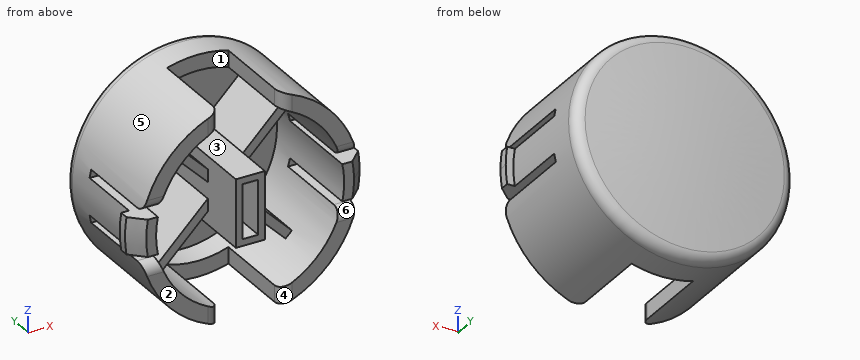
from build123d import *

# Parameters (mm, degrees)
SKETCH2_W     = 6.985
SKETCH2_H     = 32.356336156
SKETCH2_W_2   = 40.972237954
SKETCH2_H_2   = 0.889
CUTOUT_DEPTH  = 10.16
TAB_DEPTH     = 2.54
TAB_CHMF_SIZE = 1.524
CROSS_DEPTH   = 7.62
SKETCH4_W     = 3.302
SKETCH4_H     = 7.6962
BOX_DEPTH     = 13.059399
SKETCH6_W     = 1.778
SKETCH6_H     = 6.1722
BOXCUT_DEPTH  = 13.059399
FILLET1_R     = 1.27


with BuildPart() as part:
    # Sketch1 → dome/base (revolve)
    with BuildSketch(Plane.XY):
        with BuildLine():
            Line((0, 6.039891065), (0, 3.960890157))
            Line((0, 3.960890157), (10.6934, 3.960890157))
            Line((10.6934, 3.960890157), (10.6934, -9.047708935))
            Line((10.6934, -9.047708935), (12.4714, -9.047708935))
            Line((12.4714, -9.047708935), (12.4714, 4.195604597))
            ThreePointArc((12.4714, 4.195604597), (12.144228327, 5.046471653), (11.33128229, 5.45894564))
            ThreePointArc((11.33128229, 5.45894564), (5.673082405, 5.894559394), (0, 6.039891065))
        make_face()
    revolve(axis=Axis((0, 0, 0), (0, 1, 0)))

    # Sketch2 → cutout (cut)
    with BuildSketch(Plane.XZ.offset(9.047708935)):
        Rectangle(SKETCH2_W, SKETCH2_H)
        with Locations((0, 2.54)):
            Rectangle(SKETCH2_W_2, SKETCH2_H_2)
        with Locations((0, -2.54)):
            Rectangle(SKETCH2_W_2, SKETCH2_H_2)
    extrude(amount=-CUTOUT_DEPTH, mode=Mode.SUBTRACT)

    # Sketch3 → tab (add)
    with BuildSketch(Plane.XZ.offset(9.047708935)):
        with BuildLine():
            Line((-13.169324385, -2.0955), (-12.294091984, -2.0955))
            ThreePointArc((-12.294091984, -2.0955), (-12.4714, 0), (-12.294091984, 2.0955))
            Line((-12.294091984, 2.0955), (-13.169324385, 2.0955))
            ThreePointArc((-13.169324385, 2.0955), (-13.335, 0), (-13.169324385, -2.0955))
        make_face()
        with BuildLine():
            Line((12.294091984, -2.0955), (13.169324385, -2.0955))
            ThreePointArc((13.169324385, -2.0955), (13.293516571, -1.051019583), (13.335, 0))
            ThreePointArc((13.335, 0), (13.293516571, 1.051019583), (13.169324385, 2.0955))
            Line((13.169324385, 2.0955), (12.294091984, 2.0955))
            ThreePointArc((12.294091984, 2.0955), (12.4714, 0), (12.294091984, -2.0955))
        make_face()
    extrude(amount=-TAB_DEPTH)

    # tab chmf
    tab_chmf_edges = [part.edges().sort_by_distance(p)[0] for p in [
        (-13.335, -9.047708935, 0),
        (13.335, -9.047708935, 0),
    ]]
    chamfer(tab_chmf_edges, length=TAB_CHMF_SIZE)

    # Sketch5 → cross (add)
    with BuildSketch(Plane.XZ.offset(-3.960890157)):
        with BuildLine():
            Line((0, -0.71842049), (-0.71842049, 0))
            Line((-0.71842049, 0), (-7.91204877, -7.19362828))
            ThreePointArc((-7.91204877, -7.19362828), (-7.561375654, -7.561375654), (-7.19362828, -7.91204877))
            Line((-7.19362828, -7.91204877), (0, -0.71842049))
        make_face()
        with BuildLine():
            Line((7.91204877, -7.19362828), (0.71842049, 0))
            Line((0.71842049, 0), (0, -0.71842049))
            Line((0, -0.71842049), (7.19362828, -7.91204877))
            ThreePointArc((7.19362828, -7.91204877), (7.561375654, -7.561375654), (7.91204877, -7.19362828))
        make_face()
        with BuildLine():
            Line((7.19362828, 7.91204877), (0, 0.71842049))
            Line((0, 0.71842049), (0.71842049, 0))
            Line((0.71842049, 0), (7.91204877, 7.19362828))
            ThreePointArc((7.91204877, 7.19362828), (7.561375654, 7.561375654), (7.19362828, 7.91204877))
        make_face()
        Polygon((0.71842049, 0), (0, 0.71842049), (-0.71842049, 0), (0, -0.71842049), align=None)
        with BuildLine():
            Line((-0.71842049, 0), (0, 0.71842049))
            Line((0, 0.71842049), (-7.19362828, 7.91204877))
            ThreePointArc((-7.19362828, 7.91204877), (-7.561375654, 7.561375654), (-7.91204877, 7.19362828))
            Line((-7.91204877, 7.19362828), (-0.71842049, 0))
        make_face()
    extrude(amount=CROSS_DEPTH)

    # Sketch4 → box (add)
    with BuildSketch(Plane.XZ.offset(-3.960890157)):
        Rectangle(SKETCH4_W, SKETCH4_H)
    extrude(amount=BOX_DEPTH)

    # Sketch6 → boxcut (cut)
    with BuildSketch(Plane.XZ.offset(9.098508935)):
        Rectangle(SKETCH6_W, SKETCH6_H)
    extrude(amount=-BOXCUT_DEPTH, mode=Mode.SUBTRACT)

    # Fillet1
    fillet1_edges = [part.edges().sort_by_distance(p)[0] for p in [
        (-3.4925, -9.047708935, -11.039692922),
        (3.4925, -9.047708935, -11.039692922),
        (11.188751506, -9.047708935, -2.9845),
        (-11.188751506, -9.047708935, -2.9845),
        (-3.4925, -9.047708935, 11.039692922),
        (3.4925, -9.047708935, 11.039692922),
        (-11.188751506, -9.047708935, 2.9845),
        (11.188751506, -9.047708935, 2.9845),
    ]]
    fillet(fillet1_edges, radius=FILLET1_R)


solid = part.part
Could you check a few things on this model? Use its own coordinates, in mm. Face numbers are marked on the shaded views. A direction names the side the tool comes from. Coordinates: 2 decimals unless noted, no trailing zeros. Loops run counter-clockwise (first coordinate to the right, second up) from the corner with the lowest first, then second, coordinate; pieces in that order, holes last. Notation, with made-up numbers: (-30, 89) -> (9, 89) arc R27 ccw to (9, 112) -> close; hole circle Ø4 at (66, 18.5). An arc over 180 degrees is marked (long way). Answer in a Markdown table with one row per item.
(1) Thinking about a two-plate mould opening in Z: for the marked faces 4, 5 and 6, which applies, released by +Z, released by -Z, zero draft, split by the parting line, or undercut?
Results found:
| item | result |
|---|---|
| face 4 | zero draft |
| face 5 | split by the parting line |
| face 6 | undercut |
(2) Will these pins go through, and if not, where does the flat tip stop? pin 1 Ø6 at (y, z) = (-4, 8.5) entering from +X; pin 2 Ø1.9 at (y, z) = (-3, 0) entering from +X; pin 3 Ø8 at (y, z) = (-6.5, -8.5) entering from +X.
Results found:
| item | result |
|---|---|
| pin 1 | stops at x = 11.19 |
| pin 2 | stops at x = 12.47 |
| pin 3 | stops at x = 11.63 |
(3) Imagine slicing it at A-A (x = 0). List the corners of the cut face in (y, z) for me, plus the area to 3 significant figures.
Results found:
| item | result |
|---|---|
| outline | (-9.1, -3.85) -> (3.96, -3.85) -> (3.96, -10.69) -> (1.11, -10.69) -> (1.11, -12.47) -> (4.2, -12.47) arc R1.27 ccw to (5.46, -11.33) arc R110.8 ccw to (5.46, 11.33) arc R1.27 ccw to (4.2, 12.47) -> (1.11, 12.47) -> (1.11, 10.69) -> (3.96, 10.69) -> (3.96, 3.85) -> (-9.1, 3.85) -> (-9.1, 3.09) -> (3.96, 3.09) -> (3.96, -3.09) -> (-9.1, -3.09) -> close |
| area | 75.5 mm^2 |
(4) For the marked faces 1, 2 and 3, which set-ups out of +Z, -Z, +X, -X, +Y, -Y let a thin tool reach every point of the face, with its end or its side?
Results found:
| item | result |
|---|---|
| face 1 | +Z, -Y |
| face 2 | +Z, -Z, +X, -X, -Y |
| face 3 | -Y |
(5) Imagine slicing it at B-B (y = -1.25). Give the number of separate pieces and of enclosed holes in the cut face, plus the area to 3 significant figures.
Results found:
| item | result |
|---|---|
| separate pieces | 3 |
| enclosed holes | 1 |
| area | 146 mm^2 |
(6) If I drill on probe 1 along X at (y, z) = (-6, 0); probe 2 along Z at (x, y) = (0, 3.5); probe 3 along Z at (x, y) = (0, -4), over which ranges is the centre line in solid material (lowest first)?
Results found:
| item | result |
|---|---|
| probe 1 | x = -12.47 to -10.69, -1.65 to -0.89, 0.89 to 1.65, 10.69 to 12.47 |
| probe 2 | z = -12.47 to -10.69, -3.85 to -3.09, 3.09 to 3.85, 10.69 to 12.47 |
| probe 3 | z = -3.85 to -3.09, 3.09 to 3.85 |
